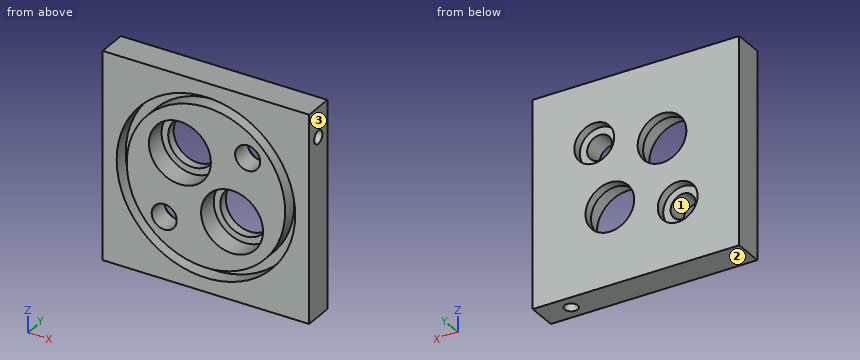
```python
from build123d import *

# Parameters (mm, degrees)
SKETCH_W            = 70
SKETCH_H            = 70
PAD_DEPTH           = 10
SKETCH001_R         = 30.25
SKETCH001_R_2       = 26.85
POCKET_DEPTH        = 5
SKETCH003_R         = 2.25
HOLE_DEPTH          = 10
HOLE_TIPS_R         = 2.25
SKETCH004_R         = 2.25
HOLE001_DEPTH       = 10
HOLE001_TIPS_R      = 2.25
HOLE003_D           = 16.5
HOLE003_CBORE_D     = 21
HOLE003_CBORE_DEPTH = 7
HOLE004_D           = 8.5
HOLE004_CBORE_D     = 13.5
HOLE004_CBORE_DEPTH = 3


with BuildPart() as part:
    # Sketch → Pad (new body)
    with BuildSketch(Plane.XZ):
        Rectangle(SKETCH_W, SKETCH_H)
    extrude(amount=PAD_DEPTH)

    # Sketch001 (on Face6 of Pad) → Pocket (cut)
    with BuildSketch(Plane.XZ.offset(10)):
        Circle(SKETCH001_R)
        Circle(SKETCH001_R_2, mode=Mode.SUBTRACT)
    extrude(amount=-POCKET_DEPTH, mode=Mode.SUBTRACT)

    # Sketch003 (on Face3 of Pocket) → Hole (cut)
    with BuildSketch(Plane(origin=(35, 0, 0), x_dir=(0, 0, 1), z_dir=(1, 0, 0))):
        with Locations((25, 5)):
            Circle(SKETCH003_R)
    extrude(amount=-HOLE_DEPTH, mode=Mode.SUBTRACT)

    # Hole tips → Hole tip 1 section 0
    with BuildSketch(Plane(origin=(25, 0, 0), x_dir=(0, 0, 1), z_dir=(1, 0, 0)), mode=Mode.PRIVATE) as hole_tip_1_s0:
        with Locations((25, 5)):
            Circle(HOLE_TIPS_R)
    loft([hole_tip_1_s0.sketch, Vertex(23.648064, -5, 25)], mode=Mode.SUBTRACT)

    # Sketch004 (on Face6 of Hole) → Hole001 (cut)
    with BuildSketch(Plane(origin=(0, 0, -35), x_dir=(1, 0, 0), z_dir=(0, 0, -1))):
        with Locations((25, 5)):
            Circle(SKETCH004_R)
    extrude(amount=-HOLE001_DEPTH, mode=Mode.SUBTRACT)

    # Hole001 tips → Hole001 tip 1 section 0
    with BuildSketch(Plane(origin=(0, 0, -25), x_dir=(1, 0, 0), z_dir=(0, 0, -1)), mode=Mode.PRIVATE) as hole001_tip_1_s0:
        with Locations((25, 5)):
            Circle(HOLE001_TIPS_R)
    loft([hole001_tip_1_s0.sketch, Vertex(25, -5, -23.648064)], mode=Mode.SUBTRACT)

    # Hole003 (through all)
    with Locations(Plane.XZ.offset(10)):
        with Locations((-8.838835, 8.838835), (8.838835, -8.838835)):
            CounterBoreHole(HOLE003_D / 2, HOLE003_CBORE_D / 2, HOLE003_CBORE_DEPTH)

    # Hole004 (through all)
    with Locations(Plane(origin=(0, 0, 0), x_dir=(1, 0, 0), z_dir=(0, 1, 0))):
        with Locations((-14.142136, 14.142136), (14.142136, -14.142136)):
            CounterBoreHole(HOLE004_D / 2, HOLE004_CBORE_D / 2, HOLE004_CBORE_DEPTH)


solid = part.part
```
Part model, mm, in its own coordinate system. Face numbers are marked on the shaded views. Round coordinates to 2 decimals unless told otherwise and drop trailing zeros. Loops run counter-clockwise (first coordinate to the right, second up) from the corner with the lowest first, then second, coordinate; pieces in that order, holes last. Notation, with made-up numbers: (78, 41.25) -> (106, 41.25) arc R17 ccw to (106, 53.25) -> close; hole circle Ø2 at (89, 35). An arc over 180 degrees is marked (long way). Use a Markdown table: item, result.
1) Cut at A-A, the plane z = 16. List the corners of the cut face in (x, y), and give its area (3 significant figures).
The answers:
| item | result |
|---|---|
| outline | (-35, -10) -> (-25.67, -10) -> (-25.67, -5) -> (-21.56, -5) -> (-21.56, -10) -> (-16.52, -10) -> (-16.52, -3) -> (-12.94, -3) -> (-12.94, 0) -> (-35, 0) -> close; (-4.74, -3) -> (-1.16, -3) -> (-1.16, -10) -> (10.32, -10) -> (10.32, -3) -> (7.65, -3) -> (7.65, 0) -> (-4.74, 0) -> close; (17.96, -10) -> (21.56, -10) -> (21.56, -5) -> (25.67, -5) -> (25.67, -10) -> (35, -10) -> (35, 0) -> (20.63, 0) -> (20.63, -3) -> (17.96, -3) -> close |
| area | 434 mm2 |
2) Probe line 1 (Z direction, x = -23, y = -6.5); line 2 (X direction, y = -7.5, z = 7); line 3 (Z direction, x = 13.5, y = -4.25). List the from-to ranges inside material, lowest first. Write a range as [from, to].
The answers:
| item | result |
|---|---|
| line 1 | z = [-35, -19.65], [-13.85, 13.85], [19.65, 35] |
| line 2 | x = [-35, -29.43], [-25.92, -19.18], [1.5, 25.92], [29.43, 35] |
| line 3 | z = [-35, -18.25], [0.57, 9.94], [18.34, 35] |
3) Pull direction Z, two halves, no side cores. Call the marked faces 1, 2 and 3: pulls with the +Z half, pulls with the -Z half, needs draft (parallel to the pull), parting line crosses it, or undercut.
The answers:
| item | result |
|---|---|
| face 1 | undercut |
| face 2 | pulls with the -Z half |
| face 3 | needs draft |
4) Drop flat-ended pins along their axis: pin 1 Ø7.5 at (x, z) = (14.14, 14.14) entering from -Y; pin 2 Ø7 at (x, z) = (16, 14) entering from +Y; pin 3 Ø6.5 at (x, z) = (-12.5, 13.5) entering from -Y. Give the stop position or say it passes through.
The answers:
| item | result |
|---|---|
| pin 1 | passes through |
| pin 2 | stops at y = -3 |
| pin 3 | stops at y = -3 |
5) Cut at B-B, the plane x = 13.5. List the corners of the cut face in (y, z).
The answers:
| item | result |
|---|---|
| outline | (-10, -35) -> (0, -35) -> (0, -15.65) -> (-3, -15.65) -> (-3, -18.25) -> (-10, -18.25) -> (-10, -23.21) -> (-5, -23.21) -> (-5, -27.07) -> (-10, -27.07) -> close; (-10, 0.57) -> (-3, 0.57) -> (-3, -2.03) -> (0, -2.03) -> (0, 7.42) -> (-3, 7.42) -> (-3, 9.94) -> (-10, 9.94) -> close; (-10, 18.34) -> (-3, 18.34) -> (-3, 20.86) -> (0, 20.86) -> (0, 35) -> (-10, 35) -> (-10, 27.07) -> (-5, 27.07) -> (-5, 23.21) -> (-10, 23.21) -> close |
6) Cut at D-D, the plane z = -26. List the corners of the cut face in (x, y).
The answers:
| item | result |
|---|---|
| outline | (-35, -10) -> (-15.46, -10) -> (-15.46, -5) -> (-6.7, -5) -> (-6.7, -10) -> (6.7, -10) -> (6.7, -5) -> (15.46, -5) -> (15.46, -10) -> (35, -10) -> (35, 0) -> (-35, 0) -> close; hole circle Ø4.5 at (25, -5) |
7) Cut at C-C, the plane y = -1. List the corners of the cut face in (x, z), and give its area (3 significant figures).
The answers:
| item | result |
|---|---|
| outline | (-35, -35) -> (35, -35) -> (35, 35) -> (-35, 35) -> close; hole circle Ø13.5 at (-14.14, -14.14); hole circle Ø16.5 at (-8.84, 8.84); hole circle Ø16.5 at (8.84, -8.84); hole circle Ø13.5 at (14.14, 14.14) |
| area | 4,190 mm2 |
